```python
from build123d import *

# Parameters (mm, degrees)
BOSS_EXTRUDE4_DEPTH            = 40
SKETCH18_R                     = 12.5
BOSS_EXTRUDE2_DEPTH            = 5
SKETCH19_R                     = 9.95
BOSS_EXTRUDE3_DEPTH            = 30
FILLET1_R                      = 10
M5_CLEARANCE_HOLE1_D           = 5.5
M5_CLEARANCE_HOLE1_CSINK_D     = 5.55
M5_CLEARANCE_HOLE1_CSINK_ANGLE = 90
CHAMFER1_SIZE                  = 1


with BuildPart() as part:
    # Sketch20 → Boss-Extrude4 (new body)
    with BuildSketch(Plane(origin=(0, 0, 0), x_dir=(1, 0, 0), z_dir=(0, 1, 0))):
        with BuildLine():
            Line((0, 0), (0, -20))
            Line((0, -20), (0, -40))
            Line((0, -40), (0.977942369, -40))
            ThreePointArc((0.977942369, -40), (60.043109857, -164.956890143), (185, -224.022057631))
            Line((185, -224.022057631), (185, -225))
            Line((185, -225), (205, -225))
            Line((205, -225), (205, -210))
            Line((205, -210), (185, -210))
            Line((185, -210), (185, -208.944436277))
            ThreePointArc((185, -208.944436277), (70.649711575, -154.350288425), (16.055563723, -40))
            Line((16.055563723, -40), (15, -40))
            Line((15, -40), (15, -20))
            Line((15, -20), (15, 0))
            Line((15, 0), (0, 0))
        make_face()
    extrude(amount=BOSS_EXTRUDE4_DEPTH)

    # Sketch18 → Boss-Extrude2 (add)
    with BuildSketch(Plane.ZY):
        with Locations((20, 20)):
            Circle(SKETCH18_R)
    extrude(amount=BOSS_EXTRUDE2_DEPTH)

    # Sketch19 → Boss-Extrude3 (add)
    with BuildSketch(Plane.ZY.offset(5)):
        with Locations((20, 20)):
            Circle(SKETCH19_R)
    extrude(amount=BOSS_EXTRUDE3_DEPTH)

    # Fillet1
    fillet1_edges = [part.edges().sort_by_distance(p)[0] for p in [
        (7.5, 0, 0),
        (7.5, 40, 0),
    ]]
    fillet(fillet1_edges, radius=FILLET1_R)

    # M5 Clearance Hole1 (through all)
    with Locations(Plane.XY.offset(225)):
        with Locations((195, 30), (195, 10)):
            CounterSinkHole(M5_CLEARANCE_HOLE1_D / 2, M5_CLEARANCE_HOLE1_CSINK_D / 2, counter_sink_angle=M5_CLEARANCE_HOLE1_CSINK_ANGLE)

    # Chamfer1
    chamfer1_edges = [part.edges().sort_by_distance(p)[0] for p in [
        (-35, 20, 10.05),
    ]]
    chamfer(chamfer1_edges, length=CHAMFER1_SIZE)


solid = part.part
```
Work out the finished part from the listing and answer in its coordinate system (mm). A direction names the side the tool comes from. Coordinates: 2 decimals unless noted, no trailing zeros. Write each loop counter-clockwise with the first axis right and the second up, starting at its lowest first coordinate (ties: lowest second). Pieces come first, ordered by that corner, then holes.
Q1. A cutting plane is placed at A-A, the plane x = 195. Give the vertices of the cut face in (y, z) (3 decimals).
Q2. Which of the six approach directions +Z, -Z, +X, -X, +Y, -Y give full straight-line access (tool end or side, diameter ignored) to faces 1 (the face through (15, 20, 20)), 2 (the face through (-2.46, 8.91, 25.77)), 3 (the face through (7.4, 3.01, 2.85))?
Q3. A cutting plane is placed at D-D, the plane x = 33.5. Give the vertices of the cut face in (y, z), then the cut area to 3 significant figures.
Q4. Each of these flat-tipped pins is pushed along its axis until it touches: pin 1 Ø0.8 at (y, z) = (20, 224.5) entering from -X; pin 2 Ø6 at (x, y) = (39, 34) entering from +Z; pin 3 Ø2 at (x, y) = (-3.5, 29) entering from -Z. Where does it stop, or does it pass through?
Q5. Find the intervals of material crossed by line 1 (Y direction, x = 195, z = 220.75); line 2 (Z direction, x = 191.5, y = 14.5); line 3 (X direction, y = 31, z = 31), in increasing order.
Q6. Determine the mould class of faces 4 (the face through (71.93, 19.72, 155.62)), 5 (the face through (192.38, 10.83, 217.38)), 6 (the face through (64, 40, 149)), 7 (the face through (192.38, 30.83, 217.38)) for opening direction X: released by +X, released by -X, zero draft, split by the parting line, or undercut.
Q7. A cutting plane is placed at C-C, the plane z = 20. Give the vertices of the cut face in (x, y), then the cut area to 3 significant figures.
Q8. A cutting plane is placed at B-B, the plane y = 20. Give the vertices of the cut face in (x, z), then the cut area to 3 significant figures.
Findings below:
1. outline: (0, 210) - (7.25, 210) - (7.25, 224.975) - (7.225, 225) - (0, 225) - close; (12.75, 210) - (27.25, 210) - (27.25, 224.975) - (27.225, 225) - (12.775, 225) - (12.75, 224.975) - close; (32.75, 210) - (40, 210) - (40, 225) - (32.775, 225) - (32.75, 224.975) - close
2. face 1: -Z, +X, +Y, -Y
2. face 2: -X
2. face 3: -Z, +X, -X, -Y
3. outline: (0, 101.78) - (40, 101.78) - (40, 132.31) - (0, 132.31) - close
3. area: 1,220 mm2
4. pin 1: stops at x = 185
4. pin 2: stops at z = 144.32
4. pin 3: stops at z = 10.4
5. line 1: y = 0 to 7.25, 12.75 to 27.25, 32.75 to 40
5. line 2: z = 210 to 225
5. line 3: x = 0 to 15
6. face 4: released by +X
6. face 5: undercut
6. face 6: zero draft
6. face 7: undercut
7. outline: (-35, 11.05) - (-34, 10.05) - (-5, 10.05) - (-5, 7.5) - (0, 7.5) - (0, 0) - (15, 0) - (15, 40) - (0, 40) - (0, 32.5) - (-5, 32.5) - (-5, 29.95) - (-34, 29.95) - (-35, 28.95) - close
7. area: 1,320 mm2
8. outline: (-35, 11.05) - (-34, 10.05) - (-5, 10.05) - (-5, 7.5) - (0, 7.5) - (0, 0) - (15, 0) - (15, 40) - (16.06, 40) arc R190 cw to (185, 208.94) - (185, 210) - (205, 210) - (205, 225) - (185, 225) - (185, 224.02) arc R205 ccw to (0.98, 40) - (0, 40) - (0, 32.5) - (-5, 32.5) - (-5, 29.95) - (-34, 29.95) - (-35, 28.95) - close
8. area: 5,670 mm2
